from build123d import *

# Parameters (mm, degrees)
SKETCH2_W           = 10.16
SKETCH2_H           = 76.2
SKETCH2_R           = 4
SKETCH2_W_2         = 50
SKETCH2_H_2         = 10.16
SKETCH2_W_3         = 11.850089675
SKETCH2_H_3         = 89.916
SKETCH2_H_4         = 10
SKETCH2_R_2         = 3.175
SKETCH2_H_5         = 63.685061478
SKETCH2_R_3         = 4.7625
SKETCH2_H_6         = 63.685061479
BOSS_EXTRUDE1_DEPTH = 10.16


with BuildPart() as part:
    # Sketch2 → Boss-Extrude1 (new body)
    with BuildSketch(Plane.XY):
        with BuildLine():
            Line((-408.300796745, 142.616356263), (-408.921789204, 152.75736057))
            Line((-408.921789204, 152.75736057), (-459.721789204, 152.75736057))
            Line((-459.721789204, 152.75736057), (-459.721789204, -230.782639429))
            ThreePointArc((-459.721789204, -230.782639429), (-437.403325931, -284.664176156), (-383.521789204, -306.982639429))
            Line((-383.521789204, -306.982639429), (-303.52, -306.982639429))
            Line((-303.52, -306.982639429), (-270.8, -306.98263943))
            Line((-270.8, -306.98263943), (-270.8, -317.14263943))
            Line((-270.8, -317.14263943), (-220, -317.14263943))
            Line((-220, -317.14263943), (-220, -306.98263943))
            Line((-220, -306.98263943), (-55.8292, -306.982639429))
            Line((-55.8292, -306.982639429), (-55.8292, -317.14263943))
            Line((-55.8292, -317.14263943), (55.8292, -317.14263943))
            Line((55.8292, -317.14263943), (55.8292, -306.982639429))
            Line((55.8292, -306.982639429), (220, -306.98263943))
            Line((220, -306.98263943), (220, -317.14263943))
            Line((220, -317.14263943), (270.8, -317.14263943))
            Line((270.8, -317.14263943), (270.8, -306.98263943))
            Line((270.8, -306.98263943), (303.52, -306.982639429))
            Line((303.52, -306.982639429), (383.521789204, -306.982639429))
            ThreePointArc((383.521789204, -306.982639429), (437.403325931, -284.664176156), (459.721789204, -230.782639429))
            Line((459.721789204, -230.782639429), (459.721789204, 152.75736057))
            Line((459.721789204, 152.75736057), (408.921789204, 152.75736057))
            Line((408.921789204, 152.75736057), (408.921789204, 142.616356263))
            Line((408.921789204, 142.616356263), (332.721789204, 142.616356263))
            Line((332.721789204, 142.616356263), (332.721789204, 152.75736057))
            Line((332.721789204, 152.75736057), (135.250547773, 152.75736057))
            Line((135.250547773, 152.75736057), (102.394461083, 316.728644457))
            Line((102.394461083, 316.728644457), (-102.394461083, 316.728644457))
            Line((-102.394461083, 316.728644457), (-135.250547773, 152.75736057))
            Line((-135.250547773, 152.75736057), (-332.100796745, 152.75736057))
            Line((-332.100796745, 152.75736057), (-332.100796745, 142.616356263))
            Line((-332.100796745, 142.616356263), (-408.300796745, 142.616356263))
        make_face()
        with Locations((-205.08, -256.782661115)):
            Rectangle(SKETCH2_W, SKETCH2_H, mode=Mode.SUBTRACT)
        with Locations((-172.69, -250.936605381)):
            Circle(SKETCH2_R, mode=Mode.SUBTRACT)
        with Locations((-117.38, -250.936605381)):
            Circle(SKETCH2_R, mode=Mode.SUBTRACT)
        with Locations((-84.92, -256.782661115)):
            Rectangle(SKETCH2_W, SKETCH2_H, mode=Mode.SUBTRACT)
        with Locations((-172.69, -220.936605381)):
            Circle(SKETCH2_R, mode=Mode.SUBTRACT)
        with BuildLine():
            ThreePointArc((-108.5, -194.170881029), (-95, -207.670881029), (-108.5, -221.170881029))
            Line((-108.5, -221.170881029), (-113.386866529, -221.170881029))
            ThreePointArc((-113.386866529, -221.170881029), (-117.38, -224.936605381), (-121.373133471, -221.170881029))
            Line((-121.373133471, -221.170881029), (-138.5, -221.170881029))
            ThreePointArc((-138.5, -221.170881029), (-152, -207.670881029), (-138.5, -194.170881029))
            Line((-138.5, -194.170881029), (-108.5, -194.170881029))
        make_face(mode=Mode.SUBTRACT)
        with Locations((-345.16, -186.334154613)):
            Rectangle(SKETCH2_W_2, SKETCH2_H_2, mode=Mode.SUBTRACT)
        with Locations((-311.557332494, -172.10863943)):
            Rectangle(SKETCH2_W_3, SKETCH2_H_3, mode=Mode.SUBTRACT)
        with Locations((-235.16, -186.254154613)):
            Rectangle(SKETCH2_W_2, SKETCH2_H_4, mode=Mode.SUBTRACT)
        with Locations((-336.55027219, -94.687385458)):
            Circle(SKETCH2_R_2, mode=Mode.SUBTRACT)
        with Locations((195.58, -147.752560311)):
            Rectangle(SKETCH2_W, SKETCH2_H_5, mode=Mode.SUBTRACT)
        with Locations((0, -78.38263943)):
            Circle(SKETCH2_R_2, mode=Mode.SUBTRACT)
        with Locations((95.25, -84.73263943)):
            Circle(SKETCH2_R_3, mode=Mode.SUBTRACT)
        with Locations((311.557332494, -172.10863943)):
            Rectangle(SKETCH2_W_3, SKETCH2_H_3, mode=Mode.SUBTRACT)
        with Locations((336.550272189, -94.687385458)):
            Circle(SKETCH2_R_2, mode=Mode.SUBTRACT)
        with Locations((-345.16, -74.366988355)):
            Rectangle(SKETCH2_W_2, SKETCH2_H_2, mode=Mode.SUBTRACT)
        Polygon((-210.16, -79.446988355), (-260.16, -79.446988355), (-260.16, -69.446988355), (-210.16, -69.446988355), (-210.16, -8.96237531), (-200, -8.96237531), (-200, -85.16237531), (-210.16, -85.16237531), align=None, mode=Mode.SUBTRACT)
        with Locations((-378.573819589, -5.78737531)):
            Circle(SKETCH2_R_2, mode=Mode.SUBTRACT)
        with Locations((-336.55027219, -5.787385458)):
            Circle(SKETCH2_R_2, mode=Mode.SUBTRACT)
        with Locations((-311.557332494, 7.72336057)):
            Rectangle(SKETCH2_W_3, SKETCH2_H_3, mode=Mode.SUBTRACT)
        with Locations((-84.92, -47.06237531)):
            Rectangle(SKETCH2_W, SKETCH2_H, mode=Mode.SUBTRACT)
        with Locations((-172.2755, 25.75736057)):
            Circle(SKETCH2_R_3, mode=Mode.SUBTRACT)
        with Locations((-81.7245, 25.75736057)):
            Circle(SKETCH2_R_3, mode=Mode.SUBTRACT)
        with Locations((-412.75027219, 83.112614542)):
            Circle(SKETCH2_R_2, mode=Mode.SUBTRACT)
        with Locations((-336.55027219, 83.112614542)):
            Circle(SKETCH2_R_2, mode=Mode.SUBTRACT)
        with Locations((-172.2755, 127.35736057)):
            Circle(SKETCH2_R_3, mode=Mode.SUBTRACT)
        with Locations((-81.7245, 127.35736057)):
            Circle(SKETCH2_R_3, mode=Mode.SUBTRACT)
        with Locations((81.7245, 25.75736057)):
            Circle(SKETCH2_R_3, mode=Mode.SUBTRACT)
        with Locations((195.58, -20.382437355)):
            Rectangle(SKETCH2_W, SKETCH2_H_6, mode=Mode.SUBTRACT)
        with Locations((172.2755, 25.75736057)):
            Circle(SKETCH2_R_3, mode=Mode.SUBTRACT)
        with Locations((311.557332494, 7.72336057)):
            Rectangle(SKETCH2_W_3, SKETCH2_H_3, mode=Mode.SUBTRACT)
        with Locations((336.550272189, -5.787385458)):
            Circle(SKETCH2_R_2, mode=Mode.SUBTRACT)
        with Locations((378.573819589, -5.78737531)):
            Circle(SKETCH2_R_2, mode=Mode.SUBTRACT)
        with Locations((81.7245, 127.35736057)):
            Circle(SKETCH2_R_3, mode=Mode.SUBTRACT)
        with Locations((195.58, 106.97026018)):
            Rectangle(SKETCH2_W, SKETCH2_H_6, mode=Mode.SUBTRACT)
        with Locations((172.2755, 127.35736057)):
            Circle(SKETCH2_R_3, mode=Mode.SUBTRACT)
        with Locations((336.550272189, 83.112614542)):
            Circle(SKETCH2_R_2, mode=Mode.SUBTRACT)
        with Locations((412.750272189, 83.112614542)):
            Circle(SKETCH2_R_2, mode=Mode.SUBTRACT)
    extrude(amount=-BOSS_EXTRUDE1_DEPTH)


solid = part.part
Verification items for the finished model (mm, model axes). Give positions to 0.01 mm unless a question says otherwise; leave off trailing zeros. Answer as a JSON object with one key per item and string values. Group by question number.
1) Scan lines: line 1 along Y through (x, z) = (-343.5, -2); line 2 along X through (y, z) = (-134, -5.25); line 3 along X through (y, z) = (19, -5.5). Record each from-to range of solid material in increasing order. Write a range as [from, to].
2) Cross-section at A-A (z = -5.25). Give the number of separate pieces and of enclosed holes in the cut face, then the cut area to 3 significant figures.
3) Depth check by flat-ended pin: pin 1 Ø1 at (x, z) = (-203, -6.5) entering from -Y; pin 2 Ø3 at (x, z) = (-207, -5) entering from +Y; pin 3 Ø1.5 at (y, z) = (-241.5, -7.5) entering from -X. Enter the tip coordinate at first touch or a pass-through.
Result sheet:
{
 "1": {"line 1": "y = [-306.98, -191.41], [-181.25, -79.45], [-69.29, 142.62]", "line 2": "x = [-459.72, -317.48], [-305.63, 190.5], [200.66, 305.63], [317.48, 459.72]", "line 3": "x = [-459.72, -317.48], [-305.63, 305.63], [317.48, 459.72]"},
 "2": {"separate pieces": "1", "enclosed holes": "38", "area": "446,000 mm2"},
 "3": {"pin 1": "stops at y = -306.98", "pin 2": "stops at y = 152.76", "pin 3": "stops at x = -459.07"}
}
